Autodesk Inventor part; units mm, degrees
ref_plane "YZ Plane" through (0, 0, 0) normal (1, 0, 0) x (0, 1, 0)
ref_plane "XZ Plane" through (0, 0, 0) normal (0, 1, 0) x (-1, 0, 0)
ref_plane "XY Plane" through (0, 0, 0) normal (0, 0, 1) x (1, 0, 0)
sketch "Sketch1" plane through (0, 0, 0) normal (0, 1, 0) x (-1, 0, 0)
  line L0 (-6.35, 6.35) -> (6.35, 6.35)
  line L1 (6.35, 6.35) -> (6.35, -6.35)
  line L2 (6.35, -6.35) -> (-6.35, -6.35)
  line L3 (-6.35, -6.35) -> (-6.35, 6.35)
  line L4 (-6.35, 6.35) -> (6.35, -6.35) construction
  line L5 (6.35, 6.35) -> (-6.35, -6.35) construction
  circle A0 centre (0, 0) radius 1.7
  dimension "d0" = 12.7
  dimension "d1" = 12.7
  dimension "d2" = 3.4
extrude "Extrusion1" add sketch "Sketch1" along normal blind 77.6732
ref_plane "Work Plane1" through (0, 74.6732, 0) normal (0, 1, 0) x (1, 0, 0)
sketch "Sketch2" plane through (0, 74.6732, 0) normal (0, 1, 0) x (1, 0, 0)
  circle A0 centre (0, 0) radius 1.7 construction
  circle A1 centre (0, 0) radius 3.45 construction
  line L0 (0, -3.45) -> (-2.9878, -1.725)
  line L1 (-2.9878, -1.725) -> (-2.9878, 6.35)
  line L2 (2.9878, 6.35) -> (2.9878, -1.725)
  line L3 (2.9878, -1.725) -> (0, -3.45)
  line L4 (6.35, 6.35) -> (-6.35, 6.35)
  line L5 (-2.9878, 6.35) -> (2.9878, 6.35)
  dimension "d6" = 6.9
extrude "Extrusion2" cut sketch "Sketch2" against normal blind 2.8
ref_plane "Work Plane2" through (0, 3, 0) normal (0, -1, 0) x (1, 0, 0)
sketch "Sketch3" plane through (0, 3, 0) normal (0, -1, 0) x (1, 0, 0)
  circle A0 centre (0, 0) radius 3.45 construction
  line L0 (2.9878, 1.725) -> (0, 3.45)
  line L1 (0, 3.45) -> (2.9878, 1.725)
  line L2 (2.9878, 1.725) -> (2.9878, -6.35)
  line L3 (-2.9878, -6.35) -> (-2.9878, 1.725)
  line L4 (-2.9878, 1.725) -> (0, 3.45)
  line L5 (6.35, -6.35) -> (-6.35, -6.35)
  line L6 (-2.9878, -6.35) -> (2.9878, -6.35)
  point P0 (2.9878, 1.725)
  dimension "d10" = 6.9
extrude "Extrusion3" cut sketch "Sketch3" against normal blind 2.8
sketch "Sketch4" plane through (6.35, 0, -6.35) normal (0, 0, -1) x (-1, 0, 0)
  line L0 (0, 0) -> (0, 77.6732)
  line L1 (12.7, 6.8) -> (0, 6.8)
  line L2 (0, 6.8) -> (0, 70.8732)
  line L3 (0, 70.8732) -> (12.7, 70.8732)
  line L4 (12.7, 70.8732) -> (12.7, 6.8)
  line L5 (9.3378, 71.8732) -> (3.3622, 71.8732)
  line L6 (3.3622, 5.8) -> (9.3378, 5.8)
  point P0 (6.35, 0)
  point P1 (0, 6.8)
  dimension "d13" = 1
  dimension "d14" = 1
extrude "Extrusion4" cut sketch "Sketch4" against normal blind 6
fillet "Fillet1" radius 1.5 4 edges at (4.0068, 6.8, -0.35) (-4.0068, 6.8, -0.35) (4.0068, 70.8732, -0.35) (-4.0068, 70.8732, -0.35)
properties part number "standoff for walls near wheel"
Input: part model. Units: mm. Frame: model coordinates. A direction names the side the tool comes from. Coordinates: 2 decimals unless noted, no trailing zeros. Loops run counter-clockwise (first coordinate to the right, second up) from the corner with the lowest first, then second, coordinate; pieces in that order, holes last. Notation, with made-up numbers: (8.5, 52.5) -> (54.5, 52.5) arc R25 ccw to (54.5, 82.5) -> close; hole circle Ø3 at (87.5, -6.5). An arc over 180 degrees is marked (long way). One line per item, written item: value.
(1) Ray query, line 1 along Y through (x, z) = (-1.75, -3); line 2 along Z through (x, y) = (0, 2.1); line 3 along Y through (x, z) = (4.25, -4.5). Return the intervals inside material, ascending.
Answer below:
line 1: y = 0 to 3, 5.8 to 6.8, 70.87 to 71.87, 74.67 to 77.67
line 2: z = -6.35 to -1.7, 1.7 to 6.35
line 3: y = 0 to 6.8, 70.87 to 77.67
(2) Cut plane A-A (z = -4.25). Output: boundary loops of the cut face in (x, y).
Answer below:
outline: (-6.35, 0) -> (6.35, 0) -> (6.35, 6.8) -> (-6.35, 6.8) -> close; (-6.35, 70.87) -> (6.35, 70.87) -> (6.35, 77.67) -> (-6.35, 77.67) -> close; hole (-2.99, 3) -> (2.99, 3) -> (2.99, 5.8) -> (-2.99, 5.8) -> close; hole (-2.99, 71.87) -> (2.99, 71.87) -> (2.99, 74.67) -> (-2.99, 74.67) -> close
(3) Cut plane B-B (y = 10). Output: boundary loops of the cut face in (x, z), then the cut area to 3 significant figures.
Answer below:
outline: (-6.35, -0.35) -> (-1.66, -0.35) arc R1.7 cw (long way) to (1.66, -0.35) -> (6.35, -0.35) -> (6.35, 6.35) -> (-6.35, 6.35) -> close
area: 79.4 mm2
(4) Draft query along X for faces 1 (the face through (-4, 39, -0.35)), 2 (the face through (-2.988, 73, -2)). Return one class per face: pulls with the +X half, pulls with the -X half, needs draft (parallel to the pull), parting line crosses it, or undercut.
Answer below:
face 1: needs draft
face 2: undercut
(5) Set-up query: faces 3 (the face through (0, 74.673, -3)), 4 (the face through (0, 6.8, -4)), 5 (the face through (0, 38, 6.35)). Return all of +Z, -Z, +X, -X, +Y, -Y with unobstructed straight access to the full face (end or side cutting, diameter ignored); none if empty.
Answer below:
face 3: -Z
face 4: -Z, +X, -X
face 5: +Z, +X, -X, +Y, -Y
(6) Cut plane C-C (x = -4.25). Output: boundary loops of the cut face in (y, z), then the cut area to 3 significant figures.
Answer below:
outline: (0, -6.35) -> (6.8, -6.35) -> (6.8, -1.85) arc R1.5 cw to (8.3, -0.35) -> (69.37, -0.35) arc R1.5 cw to (70.87, -1.85) -> (70.87, -6.35) -> (77.67, -6.35) -> (77.67, 6.35) -> (0, 6.35) -> close
area: 603 mm2
(7) Pin query (flat end, axial travel): pin 1 Ø3 at (x, y) = (2.5, 24) entering from -Z; pin 2 Ø1 at (x, y) = (-0.5, 26.5) entering from -Z. Return the tip coordinate at first contact, or that it passes through.
Answer below:
pin 1: stops at z = -0.35
pin 2: stops at z = 1.37
